```python
from build123d import *

# Parameters (mm, degrees)
SKETCH2_R           = 20
SKETCH2_R_2         = 19
BOSS_EXTRUDE1_DEPTH = 300
SKETCH3_R           = 20
BOSS_EXTRUDE2_DEPTH = 1
SKETCH2_4_R         = 23
SKETCH2_4_R_2       = 20
BOSS_EXTRUDE3_DEPTH = 15
SKETCH2_5_R         = 26
SKETCH2_5_R_2       = 25
SKETCH2_5_R_3       = 23
BOSS_EXTRUDE4_DEPTH = 2


with BuildPart() as part:
    # Sketch2 → Boss-Extrude1 (new body)
    with BuildSketch(Plane.XY):
        Circle(SKETCH2_R)
        Circle(SKETCH2_R_2, mode=Mode.SUBTRACT)
    extrude(amount=BOSS_EXTRUDE1_DEPTH)

    # Sketch3 → Boss-Extrude2 (add)
    with BuildSketch(Plane.XY.offset(300)):
        Circle(SKETCH3_R)
    extrude(amount=BOSS_EXTRUDE2_DEPTH)

    # Sketch2_4 → Boss-Extrude3 (add)
    with BuildSketch(Plane.XY):
        Circle(SKETCH2_4_R)
        Circle(SKETCH2_4_R_2, mode=Mode.SUBTRACT)
    extrude(amount=BOSS_EXTRUDE3_DEPTH)

    # Sketch2_5 → Boss-Extrude4 (add)
    with BuildSketch(Plane.XY):
        Circle(SKETCH2_5_R)
        Circle(SKETCH2_5_R_2, mode=Mode.SUBTRACT)
        Circle(SKETCH2_5_R_2)
        Circle(SKETCH2_5_R_3, mode=Mode.SUBTRACT)
    extrude(amount=BOSS_EXTRUDE4_DEPTH)


solid = part.part
```
Input: part model. Units: mm. Frame: model coordinates. A direction names the side the tool comes from. Round coordinates to 2 decimals unless told otherwise and drop trailing zeros. Loops run counter-clockwise (first coordinate to the right, second up) from the corner with the lowest first, then second, coordinate; pieces in that order, holes last.
1) Pin query (flat end, axial travel): pin 1 (4 mm diameter, centred on x = -10, z = 179, fed in from +Y); pin 2 (10 mm diameter, centred on x = -8.5, z = 71.5, fed in from -Y); pin 3 (12 mm diameter, centred on x = 18, z = 177, fed in from +Y). Return the tip coordinate at first contact, or that it passes through.
Ans:
pin 1: stops at y = 18.33
pin 2: stops at y = -19.69
pin 3: stops at y = 16
2) Pull-direction query (Y, two-part tool) for faces 3 (the flat face through (0, 0, 300)), 4 (the cylindrical face through (-4.336, -19.524, 155.998)), 5 (the flat face through (0, 0, 301)), 6 (the cylindrical face through (8.767, -16.856, 147.9)); classes: released by +Y, released by -Y, zero draft, split by the parting line, or undercut.
Ans:
face 3: undercut
face 4: split by the parting line
face 5: zero draft
face 6: undercut
3) Section query C-C on x = -14.5. Return the cut outline in (y, z), plus the area to 3 significant figures.
Ans:
outline: (-21.58, 0) - (-12.28, 0) - (-12.28, 300) - (12.28, 300) - (12.28, 0) - (21.58, 0) - (21.58, 2) - (17.85, 2) - (17.85, 15) - (13.77, 15) - (13.77, 301) - (-13.77, 301) - (-13.77, 15) - (-17.85, 15) - (-17.85, 2) - (-21.58, 2) - close
area: 1,060 mm2
4) Set-up query: faces 1 (the flat face through (10, -21, 2)), 2 (the flat face through (1.8, -19.1, 0)). Return all of +Z, -Z, +X, -X, +Y, -Y with unobstructed straight access to the full face (end or side cutting, diameter ignored); none if empty.
Ans:
face 1: +Z
face 2: -Z, +X, -X, +Y, -Y
5) Material intervals for line 1 (Y direction, x = -1.5, z = 208.5); line 2 (Y direction, x = 0, z = 175), sorted ascending.
Ans:
line 1: y = -19.94 to -18.94, 18.94 to 19.94
line 2: y = -20 to -19, 19 to 20
6) Section query B-B on y = 0. Return the cut outline in (x, z).
Ans:
outline: (-26, 0) - (-19, 0) - (-19, 300) - (19, 300) - (19, 0) - (26, 0) - (26, 2) - (23, 2) - (23, 15) - (20, 15) - (20, 301) - (-20, 301) - (-20, 15) - (-23, 15) - (-23, 2) - (-26, 2) - close
7) Section query A-A on z = 126.5. Return the cut outline in (x, y).
Ans:
outline: circle Ø40 at (0, 0); hole circle Ø38 at (0, 0)
